CAD build for the part. Positions are in the model's coordinates, mm. A direction names the side the tool comes from. Round coordinates to 2 decimals unless told otherwise and drop trailing zeros. Loops run counter-clockwise (first coordinate to the right, second up) from the corner with the lowest first, then second, coordinate; pieces in that order, holes last. Notation, with made-up numbers: (-29.75, 17) - (27.25, 17) arc R30 ccw to (27.25, 47) - close; hole circle Ø1 at (43.5, 39). An arc over 180 degrees is marked (long way). Use one line per item in the form item = value.
from build123d import *

# Parameters (mm, degrees)
F0_W     = 12
F0_H     = 12
F0_R     = 1.6
F1_DEPTH = 3
F2_DEPTH = 15
F3_R     = 1.6
F4_DEPTH = 25
F5_R     = 1.6
F6_DEPTH = 25
F9_DEPTH = 3
F10_SIZE = 3
F11_SIZE = 2


with BuildPart() as f1:
    # F0 (on Top) → F1 (new body)
    with BuildSketch(Plane.XY):
        Polygon((-40.4932990621, 0.140377609), (-55.4932990621, 0.140377609), (-55.4932990621, -14.859622391), (-52.4932990621, -14.859622391), (-52.4932990621, -2.859622391), (-40.4932990621, -2.859622391), align=None)
        with Locations((-46.4932990621, -8.859622391)):
            Rectangle(F0_W, F0_H)
        with Locations((-45.4932990621, -9.859622391)):
            Circle(F0_R, mode=Mode.SUBTRACT)
    extrude(amount=F1_DEPTH)

    # F0 (on Top) → F2 (join)
    with BuildSketch(Plane.XY):
        Polygon((-40.4932990621, 0.140377609), (-55.4932990621, 0.140377609), (-55.4932990621, -14.859622391), (-52.4932990621, -14.859622391), (-52.4932990621, -2.859622391), (-40.4932990621, -2.859622391), align=None)
    extrude(amount=F2_DEPTH)

    # F3 (on face) → F4 (cut)
    with BuildSketch(Plane(origin=(0, 0.140377609, 0), x_dir=(-1, 0, 0), z_dir=(0, 1, 0))):
        with Locations((45.4932990621, 10)):
            Circle(F3_R)
    extrude(amount=-F4_DEPTH, mode=Mode.SUBTRACT)

    # F5 (on face) → F6 (cut)
    with BuildSketch(Plane(origin=(-55.4932990621, 0, 0), x_dir=(0, -1, 0), z_dir=(-1, 0, 0))):
        with Locations((9.859622391, 10)):
            Circle(F5_R)
    extrude(amount=-F6_DEPTH, mode=Mode.SUBTRACT)

    # F8 (on 3pt) → F9 (cut)
    with BuildSketch(Plane(origin=(-7.5445588904, 7.5445588904, -7.5445588904), x_dir=(0.4082482905, 0.8164965809, 0.4082482905), z_dir=(0.5773502692, -0.5773502692, 0.5773502692))):
        Polygon((-13.727562502, 49.4428761303), (-30.1936492324, 50.4539981484), (-37.5646241009, 38.8832576573), (-31.7441225052, 25.3719072789), (-16.306232661, 24.6546380222), (-6.8639284, 39.3281951547), align=None)
    extrude(amount=-F9_DEPTH, mode=Mode.SUBTRACT)

    # F10
    f10_edges = [f1.edges().sort_by_distance(p)[0] for p in [
        (-55.493299, -7.359622, 0),
        (-47.993299, 0.140378, 0),
        (-55.493299, 0.140378, 7.5),
        (-52.493299, -8.859622, 3),
        (-46.493299, -2.859622, 3),
        (-52.493299, -2.859622, 9),
    ]]
    chamfer(f10_edges, length=F10_SIZE)

    # F11 (call 1 of 3: OpenCascade refuses the feature's edges together)
    f11_edges = [f1.edges().sort_by_distance(p)[0] for p in [
        (-40.493299, 0.140378, 7.901924),
        (-40.493299, -7.761546, 0),
        (-40.493299, -1.359622, 1.5),
    ]]
    chamfer(f11_edges, length=F11_SIZE)

    # F11#2 (call 2 of 3)
    f11_2_edges = [f1.edges().sort_by_distance(p)[0] for p in [
        (-47.591375, -14.859622, 0),
        (-55.493299, -14.859622, 7.901924),
        (-53.993299, -14.859622, 1.5),
    ]]
    chamfer(f11_2_edges, length=F11_SIZE)

    # F11#3 (call 3 of 3)
    f11_3_edges = [f1.edges().sort_by_distance(p)[0] for p in [
        (-53.993299, -1.359622, 15),
        (-55.493299, -7.761546, 15),
        (-47.591375, 0.140378, 15),
    ]]
    chamfer(f11_3_edges, length=F11_SIZE)


solid = f1.part
1) Flat gauge pins, fed straight in: pin 1 (4.5 mm diameter, centred on y = -8.5, z = 8.5, fed in from +X); pin 2 (1.5 mm diameter, centred on x = -44.5, y = -11, fed in from -Z); pin 3 (1.5 mm diameter, centred on x = -47, y = -10.5, fed in from +Z); pin 4 (8 mm diameter, centred on y = -7, z = 11.5, fed in from +X). Where does each tip first touch, or does it go through?
Report:
pin_1 = -52.49
pin_2 = 0
pin_3 = 3
pin_4 = -49.63
2) Drill centre lines: probe 1 along X at (y, z) = (-6.5, 8.75); probe 2 along Z at (x, y) = (-43.5, -11.5); probe 3 along Z at (x, y) = (-53, -12). Where is each one in solid material? Low to high.
Report:
probe_1 = -55.49 to -52.49
probe_2 = 0 to 3
probe_3 = 0.51 to 13.17
3) Tool access for faces 5 (the flat face through (-55.493, -8, 8)), 6 (the flat face through (-51.014, -10.297, 4.521)): list every direction of +Z, -Z, +X, -X, +Y, -Y with a clear straight run to the whole face (end or side of a thin tool).
Report:
face_5 = +Z, -Z, -X, +Y, -Y
face_6 = +Z, +X, -Y
4) Two-plate mould, pull along X, no slides. Class faces 1 (the flat face through (-47.42, -1.38, 1.48)), 2 (the flat face through (-51.014, -4.381, 10.437)), 3 (the cylindrical face through (-44.22, -1.34, 9.03)), 4 (the flat face through (-54.014, -1.381, 7.93)): +X half, -X half, draft (parallel to the pull), parting line (faces both ways), or undercut.
Report:
face_1 = draft
face_2 = +X half
face_3 = undercut
face_4 = -X half
5) Slice it at A-A (z = 6.5). Write the cut outline in (x, y), plus the area to 3 significant figures.
Report:
outline = (-55.49, -12.86) - (-53.49, -14.86) - (-52.49, -14.86) - (-52.49, -5.86) - (-49.49, -2.86) - (-40.49, -2.86) - (-40.49, -1.86) - (-42.49, 0.14) - (-52.49, 0.14) - (-55.49, -2.86) - close
area = 77.0 mm^2
6) Slice it at C-C (x = -53.75). Write the cut outline in (y, z), plus the area to 3 significant figures.
Report:
outline = (-14.6, 3.72) - (-12.86, 1.26) - (-2.86, 1.26) - (-1.12, 3) - (-1.12, 13) - (-3.58, 14.74) - (-11.18, 14.74) - (-14.6, 11.32) - close; hole circle Ø3.2 at (-9.86, 10)
area = 162 mm^2
7) Slice it at B-B (x = -48.75). Write the cut outline in (y, z).
Report:
outline = (-14.86, 2) - (-12.86, 0) - (-2.86, 0) - (0.14, 3) - (0.14, 13) - (-1.86, 15) - (-2.86, 15) - (-2.86, 6) - (-5.86, 3) - (-14.86, 3) - close
